from build123d import *

# Parameters (mm, degrees)
SKETCH1_R           = 25
SKETCH1_R_2         = 1.5
BOSS_EXTRUDE1_DEPTH = 7
CUT_EXTRUDE1_START  = -3
SKETCH2_R           = 2.66
SKETCH2_R_2         = 1.5
CUT_EXTRUDE1_DEPTH  = 3
BOSS_EXTRUDE2_START = -3
SKETCH3_R           = 32.5
SKETCH3_R_2         = 1.5
BOSS_EXTRUDE2_DEPTH = 3
SKETCH4_R           = 2.5
BOSS_EXTRUDE3_DEPTH = 14


with BuildPart() as part:
    # Sketch1 → Boss-Extrude1 (new body)
    with BuildSketch(Plane(origin=(0, 0, 0), x_dir=(1, 0, 0), z_dir=(0, 1, 0))):
        with Locations(Location((0, 0, 0), (0, 0, 270))):
            Circle(SKETCH1_R)
        with Locations(Location((0, 20, 0), (0, 0, 270))):
            Circle(SKETCH1_R_2, mode=Mode.SUBTRACT)
        with Locations(Location((20, 0, 0), (0, 0, 270))):
            Circle(SKETCH1_R_2, mode=Mode.SUBTRACT)
        with Locations(Location((0, -20, 0), (0, 0, 270))):
            Circle(SKETCH1_R_2, mode=Mode.SUBTRACT)
        with Locations(Location((-20, 0, 0), (0, 0, 270))):
            Circle(SKETCH1_R_2, mode=Mode.SUBTRACT)
    extrude(amount=BOSS_EXTRUDE1_DEPTH)

    # Sketch2 → Cut-Extrude1 (cut)
    # profile 1 of 4: a face of its own
    with BuildSketch(Plane(origin=(0, 7, 0), x_dir=(1, 0, 0), z_dir=(0, 1, 0)).offset(CUT_EXTRUDE1_START)):
        with Locations(Location((-20, 0, 0), (0, 0, 270))):
            Circle(SKETCH2_R)
        with Locations(Location((-20, 0, 0), (0, 0, 270))):
            Circle(SKETCH2_R_2, mode=Mode.SUBTRACT)
    # profile 2 of 4: a face of its own
    with BuildSketch(Plane(origin=(0, 7, 0), x_dir=(1, 0, 0), z_dir=(0, 1, 0)).offset(CUT_EXTRUDE1_START)):
        with Locations(Location((0, 20, 0), (0, 0, 270))):
            Circle(SKETCH2_R)
        with Locations(Location((0, 20, 0), (0, 0, 270))):
            Circle(SKETCH2_R_2, mode=Mode.SUBTRACT)
    # profile 3 of 4: a face of its own
    with BuildSketch(Plane(origin=(0, 7, 0), x_dir=(1, 0, 0), z_dir=(0, 1, 0)).offset(CUT_EXTRUDE1_START)):
        with Locations(Location((20, 0, 0), (0, 0, 270))):
            Circle(SKETCH2_R)
        with Locations(Location((20, 0, 0), (0, 0, 270))):
            Circle(SKETCH2_R_2, mode=Mode.SUBTRACT)
    # profile 4 of 4: a face of its own
    with BuildSketch(Plane(origin=(0, 7, 0), x_dir=(1, 0, 0), z_dir=(0, 1, 0)).offset(CUT_EXTRUDE1_START)):
        with Locations(Location((0, -20, 0), (0, 0, 270))):
            Circle(SKETCH2_R)
        with Locations(Location((0, -20, 0), (0, 0, 270))):
            Circle(SKETCH2_R_2, mode=Mode.SUBTRACT)
    extrude(amount=CUT_EXTRUDE1_DEPTH, mode=Mode.SUBTRACT)

    # Sketch3 → Boss-Extrude2 (add)
    with BuildSketch(Plane(origin=(0, 0, 0), x_dir=(1, 0, 0), z_dir=(0, 1, 0)).offset(BOSS_EXTRUDE2_START)):
        with Locations(Location((0, 0, 0), (0, 0, 270))):
            Circle(SKETCH3_R)
        with Locations(Location((0, 20, 0), (0, 0, 270))):
            Circle(SKETCH3_R_2, mode=Mode.SUBTRACT)
        with Locations(Location((-20, 0, 0), (0, 0, 270))):
            Circle(SKETCH3_R_2, mode=Mode.SUBTRACT)
        with Locations(Location((0, -20, 0), (0, 0, 270))):
            Circle(SKETCH3_R_2, mode=Mode.SUBTRACT)
        with Locations(Location((20, 0, 0), (0, 0, 270))):
            Circle(SKETCH3_R_2, mode=Mode.SUBTRACT)
    extrude(amount=BOSS_EXTRUDE2_DEPTH)

    # Sketch4 → Boss-Extrude3 (add)
    with BuildSketch(Plane(origin=(0, 7, 0), x_dir=(1, 0, 0), z_dir=(0, 1, 0))):
        with Locations(Location((0, 0, 0), (0, 0, 270))):
            Circle(SKETCH4_R)
    extrude(amount=BOSS_EXTRUDE3_DEPTH)


solid = part.part
CAD build for the part. Positions are in the model's coordinates, mm. A direction names the side the tool comes from. Round coordinates to 2 decimals unless told otherwise and drop trailing zeros. Order: outer loops, then holes, each group sorted by start corner. A loop starts at its lowest first (then second) coordinate and runs counter-clockwise, first axis right, second up. Notation, with made-up numbers: (20, 18.25) -> (27, 18.25) arc R34 cw to (27, 49.25) -> close; hole circle Ø5 at (-4.5, 62.5). An arc over 180 degrees is marked (long way). Write each question's results on one line, items separated by ' | '.
1. Pull direction X, two halves, no side cores. Call faces 1 (the face through (-22.597, 5.479, -0.577)), 2 (the face through (-2.44, 13.9, -0.54)), 3 (the face through (0.07, 0.45, -21.5)), 4 (the face through (-19, 0, 17)): pulls with the +X half, pulls with the -X half, needs draft (parallel to the pull), parting line crosses it, or undercut.
Findings below:
face 1: undercut | face 2: parting line crosses it | face 3: undercut | face 4: needs draft
2. Cut at B-B (x = 20). Give the cut face in (y, z), plus the area to 3 significant figures.
Findings below:
outline: (-3, -25.62) -> (0, -25.62) -> (0, -15) -> (7, -15) -> (7, -2.66) -> (4, -2.66) -> (4, -1.5) -> (-3, -1.5) -> close; (-3, 1.5) -> (4, 1.5) -> (4, 2.66) -> (7, 2.66) -> (7, 15) -> (0, 15) -> (0, 25.62) -> (-3, 25.62) -> close | area: 327 mm²
3. Cut at A-A (z = 0). Give the cut face in (x, y), plus the area to 3 significant figures.
Findings below:
outline: (-32.5, -3) -> (-21.5, -3) -> (-21.5, 4) -> (-22.66, 4) -> (-22.66, 7) -> (-25, 7) -> (-25, 0) -> (-32.5, 0) -> close; (-18.5, -3) -> (18.5, -3) -> (18.5, 4) -> (17.34, 4) -> (17.34, 7) -> (2.5, 7) -> (2.5, 21) -> (-2.5, 21) -> (-2.5, 7) -> (-17.34, 7) -> (-17.34, 4) -> (-18.5, 4) -> close; (21.5, -3) -> (32.5, -3) -> (32.5, 0) -> (25, 0) -> (25, 7) -> (22.66, 7) -> (22.66, 4) -> (21.5, 4) -> close | area: 541 mm²
4. Flat gauge pins, fed straight in: P1, Ø3.5, axis at x = 20, z = 0, coming from the +Y side; P2, Ø4.5, axis at x = 20, z = 0, coming from the -Y side; P3, Ø5, axis at y = 18.5, z = -2.5, coming from the -X side; P4, Ø5, axis at x = -14, y = 10.5, coming from the +Z side. Where does each tip first touch, or does it go through?
Findings below:
P1: stops at y = 4 | P2: stops at y = -3 | P3: stops at x = -2.5 | P4: passes through
5. Cut at D-D (y = 19.25). Give the cut face in (x, z), plus the area to 3 significant figures.
Findings below:
outline: circle Ø5 at (0, 0) | area: 19.6 mm²
6. Wall check: line 1 along X through (y, z) = (-0.5, 0); line 2 along X through (y, z) = (1, 0); line 3 along Y through (x, z) = (-21, -14.5). Give the ranges that are in metal, low to high. Write a range as [from, to].
Findings below:
line 1: x = [-32.5, -21.5], [-18.5, 18.5], [21.5, 32.5] | line 2: x = [-25, -21.5], [-18.5, 18.5], [21.5, 25] | line 3: y = [-3, 0]
7. 3-axis set-ups, long thin cutter, end or side, ignore diameter. For faces 5 (the face through (-2, 4, -20)), 6 (the face through (-18.735, 0.451, 0.806)): which of +Z, -Z, +X, -X, +Y, -Y reach the whole face in a straight line?
Findings below:
face 5: +Y | face 6: +Y, -Y
8. Cut at C-C (z = -20). Give the cut face in (x, y), plus the area to 3 significant figures.
Findings below:
outline: (-25.62, -3) -> (-1.5, -3) -> (-1.5, 4) -> (-2.66, 4) -> (-2.66, 7) -> (-15, 7) -> (-15, 0) -> (-25.62, 0) -> close; (1.5, -3) -> (25.62, -3) -> (25.62, 0) -> (15, 0) -> (15, 7) -> (2.66, 7) -> (2.66, 4) -> (1.5, 4) -> close | area: 327 mm²
